```python
from build123d import *

# Parameters (mm, degrees)
SKETCH3_R           = 2.5
SKETCH3_R_2         = 2
SKETCH5_R           = 2.5
SKETCH5_R_2         = 2
BOSS_EXTRUDE2_DEPTH = 20


with BuildPart() as part:
    # Sweep1: sweep along a path in Sketch2
    with BuildLine(Plane(origin=(0, 0, 0), x_dir=(1, 0, 0), z_dir=(0, 1, 0))) as sweep1_path:
        Line((-41, 0), (-41, -20))
        ThreePointArc((-41, -20), (-38.071067812, -27.071067812), (-31, -30))
        Line((-31, -30), (31, -30))
        ThreePointArc((31, -30), (38.071067812, -27.071067812), (41, -20))
        Line((41, -20), (41, 0))
    # Sketch3 → Sweep1 (sweep)
    with BuildSketch(Plane.XY):
        with Locations((-41, 0)):
            Circle(SKETCH3_R)
        with Locations((-41, 0)):
            Circle(SKETCH3_R_2, mode=Mode.SUBTRACT)
    sweep(path=sweep1_path.line)

    # Sketch5 → Boss-Extrude2 (add)
    with BuildSketch(Plane.XY.offset(30)):
        Circle(SKETCH5_R)
        with Locations(Location((0, 0, 0), (0, 0, 180))):
            Circle(SKETCH5_R_2, mode=Mode.SUBTRACT)
    extrude(amount=BOSS_EXTRUDE2_DEPTH)


solid = part.part
```
Verification items for the finished model (mm, model axes). A direction names the side the tool comes from. Round coordinates to 2 decimals unless told otherwise and drop trailing zeros. Write each loop counter-clockwise with the first axis right and the second up, starting at its lowest first coordinate (ties: lowest second). Pieces come first, ordered by that corner, then holes. Notation, with made-up numbers: (41, 27) -> (73, 27) arc R30 ccw to (73, 64) -> close; hole circle Ø9 at (-4.75, 53.25). An arc over 180 degrees is marked (long way). Write each question's results on one line, items separated by ' | '. Start each with the question number.
1. Set-up check for faces 5 (the flat face through (-42, 2, 0)), 6 (the cylindrical face through (-38.69, -0.96, 10.14)), 7 (the flat face through (2.2, -0.1, 30)), 8 (the cylindrical face through (0, 2, 41)): record each of +Z, -Z, +X, -X, +Y, -Y from which the full face is reachable in a straight line by a thin tool's end or side.
2. Depth check by flat-ended pin: P1, Ø3, axis at x = 1.5, y = 0, coming from the -Z side; P2, Ø3, axis at x = 0, y = 0, coming from the +Z side. Enter the tip coordinate at first touch or a pass-through.
3. Cross-section at A-A (x = 15). Enter the section's corners in (y, z), then the cut area to 3 significant figures.
4. Material ranges on probe 1 along Z at (x, y) = (6, 0); probe 2 along X at (y, z) = (0.05, 38), recorded low to high. Write a range as from..to.
5. Draft check along X on faces 1 (the cylindrical face through (-2.5, 0.1, 39.9)), 2 (the flat face through (-2.2, 0, 30)), 3 (the flat face through (42, 2, 0)), 4 (the cylindrical face through (0.434, 0.751, 27.615)). Enter one of: +X half, -X half, draft (parallel to the pull), parting line (faces both ways), or undercut.
Solutions:
1) face 5: -Z, +X, -X, +Y, -Y | face 6: -Z | face 7: none | face 8: +Z
2) P1: stops at z = 27.5 | P2: stops at z = 32.5
3) outline: circle Ø5 at (0, 30); hole circle Ø4 at (0, 30) | area: 7.07 mm2
4) probe 1: z = 27.5..28, 32..32.5 | probe 2: x = -2.5..-2, 2..2.5
5) face 1: parting line | face 2: undercut | face 3: draft | face 4: undercut
